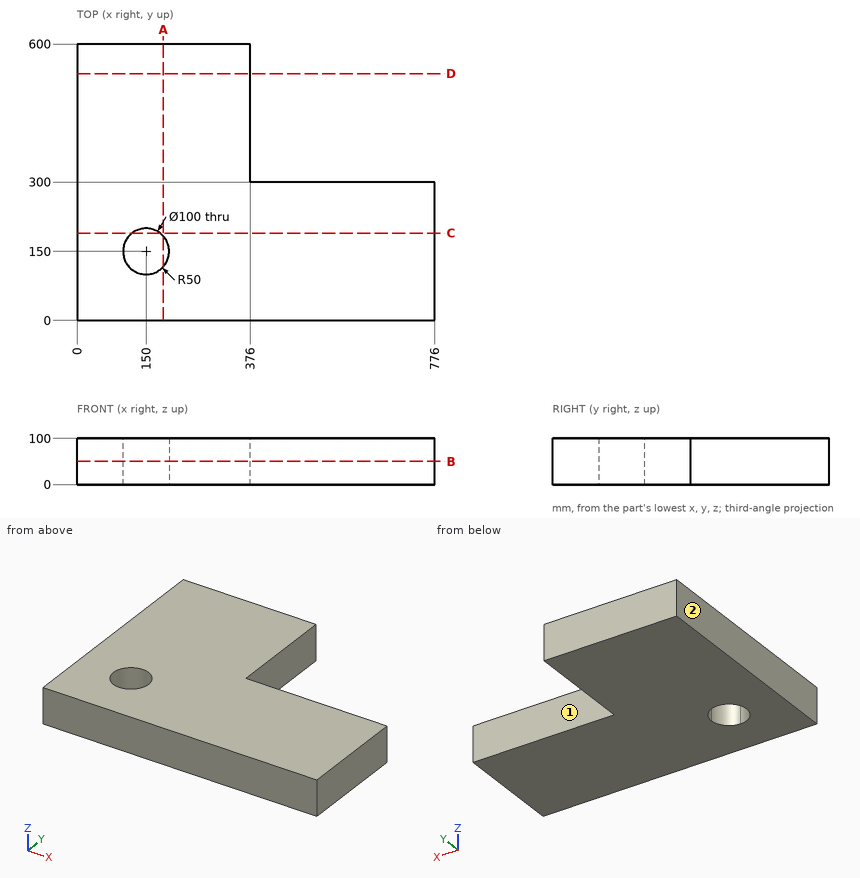
The figure shows three views and two pictorial views of one solid part (mm, origin at its lowest corner). Answer the questions. A direction names the side the tool comes from. Round coordinates to 2 decimals unless told otherwise and drop trailing zeros. Write each loop counter-clockwise with the first axis right and the second up, starting at its lowest first coordinate (ties: lowest second). Pieces come first, ordered by that corner, then holes. Notation, with made-up numbers: (37.25, 65.25) -> (82.25, 65.25) arc R30 ccw to (82.25, 94.25) -> close; hole circle Ø10 at (57, 44.25). An arc over 180 degrees is marked (long way). Answer as a JSON object with one key per item and string values. Group by question number.
Q1. Straight lines are drawn through the part: line 1 along Y through (x, z) = (150, 80); line 2 along X through (y, z) = (150, 78); line 3 along X through (y, z) = (428, 6). For each, find the intervals that lie inside material, in ascending order.
Q2. Each of these flat-tipped pins is pushed along its axis until it touches: pin 1 Ø5 at (x, y) = (538.5, 228.5) entering from -Z; pin 2 Ø6 at (y, z) = (380.5, 24) entering from +X; pin 3 Ø1 at (x, z) = (608.5, 54) entering from +Y. Where does it stop, or does it pass through?
Q3. Section A-A (x = 187.5) is taken. Write down the section's boundary in (y, z).
Q4. Which of the six approach directions +Z, -Z, +X, -X, +Y, -Y give full straight-line access (tool end or side, diameter ignored) to the marked faces 1 and 2?
Q5. Section D-D (y = 535.5) is taken. Write down the section's boundary in (x, z), plus the area to 3 significant figures.
Q6. Section C-C (y = 189.5) is taken. Write down the section's boundary in (x, z).
Q7. Section B-B (z = 50) is taken. Write down the section's boundary in (x, y).
Check values:
{
 "1": {"line 1": "0 to 100, 200 to 600", "line 2": "0 to 100, 200 to 776", "line 3": "0 to 376"},
 "2": {"pin 1": "z = 0", "pin 2": "x = 376", "pin 3": "y = 300"},
 "3": {"outline": "(0, 0) -> (116.93, 0) -> (116.93, 100) -> (0, 100) -> close; (183.07, 0) -> (600, 0) -> (600, 100) -> (183.07, 100) -> close"},
 "4": {"face 1": "+Z, -Z, +X, +Y", "face 2": "+Z, -Z, -X, +Y, -Y"},
 "5": {"outline": "(0, 0) -> (376, 0) -> (376, 100) -> (0, 100) -> close", "area": "37,600 mm^2"},
 "6": {"outline": "(0, 0) -> (119.34, 0) -> (119.34, 100) -> (0, 100) -> close; (180.66, 0) -> (776, 0) -> (776, 100) -> (180.66, 100) -> close"},
 "7": {"outline": "(0, 0) -> (776, 0) -> (776, 300) -> (376, 300) -> (376, 600) -> (0, 600) -> close; hole circle Ø100 at (150, 150)"}
}
